from build123d import *

# Parameters (mm, degrees)
F0_W     = 50.8
F0_H     = 50.8
F1_DEPTH = 3
F2_R     = 1.5
F3_DEPTH = 10
F4_R     = 12.7
F5_DEPTH = 25.4


with BuildPart() as f1:
    # F0 (on Top) → F1 (new body)
    with BuildSketch(Plane.XY):
        Rectangle(F0_W, F0_H)
    extrude(amount=F1_DEPTH)

    # F2 (on Top) → F3 (join)
    with BuildSketch(Plane.XY):
        with Locations((-12.727922, 12.727922)):
            Circle(F2_R)
        with Locations((-12.727922, -12.727922)):
            Circle(F2_R)
        with Locations((12.727922, -12.727922)):
            Circle(F2_R)
        with Locations((12.727922, 12.727922)):
            Circle(F2_R)
    extrude(amount=F3_DEPTH)

    # F4 (on face) → F5 (cut)
    with BuildSketch(Plane.XY.offset(3)):
        Circle(F4_R)
    extrude(amount=-F5_DEPTH, mode=Mode.SUBTRACT)


solid = f1.part
Part model, mm, in its own coordinate system. A direction names the side the tool comes from. Give positions to 0.01 mm unless a question says otherwise; leave off trailing zeros. Order: outer loops, then holes, each group sorted by start corner. A loop starts at its lowest first (then second) coordinate and runs counter-clockwise, first axis right, second up. Notation, with made-up numbers: (66.25, -11) -> (110.25, -11) arc R25 ccw to (110.25, 1) -> close; hole circle Ø5 at (87, 72). An arc over 180 degrees is marked (long way). Use one line per item in the form item = value.
(1) Pull direction Y, two halves, no side cores. Call faces 1 (the face through (0, -25.4, 1)), 2 (the face through (-2.75, -12.4, 1.52)), 3 (the face through (-13, -13, 10)): +Y half, -Y half, draft (parallel to the pull), parting line (faces both ways), or undercut.
Solution:
face_1 = -Y half
face_2 = undercut
face_3 = draft
(2) Saw through at C-C (z = 2). Write the cut outline in (x, y), then the cut area to 3 significant figures.
Solution:
outline = (-25.4, -25.4) -> (25.4, -25.4) -> (25.4, 25.4) -> (-25.4, 25.4) -> close; hole circle Ø25.4 at (0, 0)
area = 2,070 mm²
(3) Drill centre lines: line 1 (Y direction, x = 0, z = 0.85); line 2 (Z direction, x = 6, y = 23); line 3 (X direction, y = -12.5, z = 7.5). Where is each one in solid material? Low to high. Write a range as from..to.
Solution:
line_1 = -25.4..-12.7, 12.7..25.4
line_2 = 0..3
line_3 = -14.21..-11.25, 11.25..14.21
(4) Saw through at D-D (y = 18.5). Write the cut outline in (x, z), then the cut area to 3 significant figures.
Solution:
outline = (-25.4, 0) -> (25.4, 0) -> (25.4, 3) -> (-25.4, 3) -> close
area = 152 mm²
(5) Flat gauge pin, fed straight in: P1, Ø6, axis at x = 15.5, z = 8, coming from the +Y side. Where does the tip first touch, or does it go through?
Solution:
P1 = 14.23
(6) Tool access for faces 4 (the face through (-13, 13, 10)), 5 (the face through (-14.226, -12.662, 6.451)): list every direction of +Z, -Z, +X, -X, +Y, -Y with a clear straight run to the whole face (end or side of a thin tool).
Solution:
face_4 = +Z, +X, -X, +Y, -Y
face_5 = +Z
(7) Saw through at A-A (y = 0). Write the cut outline in (x, z).
Solution:
outline = (-25.4, 0) -> (-12.7, 0) -> (-12.7, 3) -> (-25.4, 3) -> close; (12.7, 0) -> (25.4, 0) -> (25.4, 3) -> (12.7, 3) -> close
